from build123d import *

# Parameters (mm, degrees)
EXTRUDE_THIN1_DEPTH     = 101.6
FILLET1_R               = 25.4
FILLET2_R               = 25.4
CUT_EXTRUDE1_DEPTH      = 10.922
CUT_EXTRUDE1_DEPTH_BACK = 54.61


with BuildPart() as part:
    # Sketch1 → Extrude-Thin1 (new, symmetric)
    with BuildSketch(Plane.XY):
        with BuildLine():
            Line((0, 0), (0, 5.08))
            ThreePointArc((0, 5.08), (-3.719743879, 14.060256121), (-12.7, 17.78))
            ThreePointArc((-12.7, 17.78), (-30.660512242, 25.219487758), (-38.1, 43.18))
            Line((-38.1, 43.18), (-38.1, 360.68))
            Line((-38.1, 360.68), (-30.48, 360.68))
            Line((-30.48, 360.68), (-30.48, 43.18))
            ThreePointArc((-30.48, 43.18), (-25.272358569, 30.607641431), (-12.7, 25.4))
            ThreePointArc((-12.7, 25.4), (1.668409794, 19.448409794), (7.62, 5.08))
            Line((7.62, 5.08), (7.62, 0))
            Line((7.62, 0), (0, 0))
        make_face()
    extrude(amount=EXTRUDE_THIN1_DEPTH, both=True)

    # Fillet1
    fillet1_edges = [part.edges().sort_by_distance(p)[0] for p in [
        (-34.29, 360.68, 101.6),
    ]]
    fillet(fillet1_edges, radius=FILLET1_R)

    # Fillet2
    fillet2_edges = [part.edges().sort_by_distance(p)[0] for p in [
        (-34.29, 360.68, -101.6),
    ]]
    fillet(fillet2_edges, radius=FILLET2_R)

    # Sketch3 → Cut-Extrude1 (cut, two sides: drawn at the far end of the back side and taken through both)
    with BuildSketch(Plane(origin=(7.62, 0, 0), x_dir=(0, 0, -1), z_dir=(1, 0, 0)).offset(-CUT_EXTRUDE1_DEPTH_BACK)):
        with BuildLine():
            Line((-101.6, 0), (-101.6, 63.533291796))
            ThreePointArc((-101.6, 63.533291796), (-82.785279567, 34.211252412), (-76.2, 0))
            Line((-76.2, 0), (-101.6, 0))
        make_face()
        with BuildLine():
            Line((101.6, 0), (76.2, 0))
            ThreePointArc((76.2, 0), (82.785279567, 34.211252412), (101.6, 63.533291796))
            Line((101.6, 63.533291796), (101.6, 0))
        make_face()
    extrude(amount=CUT_EXTRUDE1_DEPTH + CUT_EXTRUDE1_DEPTH_BACK, mode=Mode.SUBTRACT)


solid = part.part
Verification items for the finished model (mm, model axes). A direction names the side the tool comes from. Give positions to 0.01 mm unless a question says otherwise; leave off trailing zeros. Loops run counter-clockwise (first coordinate to the right, second up) from the corner with the lowest first, then second, coordinate; pieces in that order, holes last.
1) Thickness scan on line 1 along X through (y, z) = (304, -9.5); line 2 along Y through (x, z) = (-12.5, 76.5); line 3 along Y through (x, z) = (2, 46). Record the ranges inside material, lowest first.
2) Sectioned sample at B-B, the plane y = 224.5. Enter the section's corners in (x, z), then the cut area to 3 significant figures.
3) Sectioned sample at A-A, the plane z = 31. Enter the section's corners in (x, y).
4) Sectioned sample at C-C, the plane x = -16.5. Enter the section's corners in (y, z).
5) Depth check by flat-ended pin: pin 1 Ø8 at (x, z) = (-26.5, -64.5) entering from -Y; pin 2 Ø2 at (x, z) = (-33, 32) entering from -Y; pin 3 Ø1.5 at (y, z) = (3, -15) entering from -X. Enter the tip coordinate at first touch or a pass-through.
6) Set-up check for faces 1 (the flat face through (-30.48, 204, 1)), 2 (the flat face through (-34, 201, 101.6)): record each of +Z, -Z, +X, -X, +Y, -Y from which the full face is reachable in a straight line by a thin tool's end or side.
Answers:
1. line 1: x = -38.1 to -30.48
1. line 2: y = 17.78 to 25.4
1. line 3: y = 0 to 19.11
2. outline: (-38.1, -101.6) - (-30.48, -101.6) - (-30.48, 101.6) - (-38.1, 101.6) - close
2. area: 1,550 mm2
3. outline: (-38.1, 43.18) arc R25.4 ccw to (-12.7, 17.78) arc R12.7 cw to (0, 5.08) - (0, 0) - (7.62, 0) - (7.62, 5.08) arc R20.32 ccw to (-12.7, 25.4) arc R17.78 cw to (-30.48, 43.18) - (-30.48, 360.68) - (-38.1, 360.68) - close
4. outline: (18.07, -77.99) arc R92.16 cw to (25.81, -79.89) - (25.81, 79.89) arc R92.16 cw to (18.07, 77.99) - close
5. pin 1: stops at y = 19.75
5. pin 2: stops at y = 26.67
5. pin 3: stops at x = 0
6. face 1: +Z, -Z, +X, +Y
6. face 2: +Z, +X, -X, +Y, -Y
